from build123d import *

# Parameters (mm, degrees)
SKETCH1_R           = 53.975
SKETCH1_R_2         = 49.975
BOSS_EXTRUDE1_DEPTH = 283.75
SKETCH2_R           = 53.975
BOSS_EXTRUDE2_DEPTH = 4
FILLET1_R           = 5


with BuildPart() as part:
    # Sketch1 → Boss-Extrude1 (new, symmetric)
    with BuildSketch(Plane(origin=(0, 0, 0), x_dir=(1, 0, 0), z_dir=(0, 1, 0))):
        with Locations(Location((0, 0, 0), (0, 0, 270))):
            Circle(SKETCH1_R)
        with Locations(Location((0, 0, 0), (0, 0, 270))):
            Circle(SKETCH1_R_2, mode=Mode.SUBTRACT)
    extrude(amount=BOSS_EXTRUDE1_DEPTH, both=True)

    # Sketch2 → Boss-Extrude2 (add)
    with BuildSketch(Plane.XZ.offset(283.75)):
        with Locations(Location((0, 0, 0), (0, 0, 270))):
            Circle(SKETCH2_R)
    extrude(amount=BOSS_EXTRUDE2_DEPTH)

    # Sketch3 → Revolve1 (revolve)
    with BuildSketch(Plane.XY, mode=Mode.PRIVATE) as revolve1_sk:
        with BuildLine():
            Line((-14.520190182, 339.3125), (-14.520190182, 361.5375))
            Line((-14.520190182, 361.5375), (-10.520190182, 361.5375))
            Line((-10.520190182, 361.5375), (-10.520190182, 336.395540435))
            ThreePointArc((-10.520190182, 336.395540435), (-39.016633765, 316.644661214), (-49.975, 283.75))
            Line((-49.975, 283.75), (-53.975, 283.75))
            ThreePointArc((-53.975, 283.75), (-43.107974032, 317.822985722), (-14.520190182, 339.3125))
        make_face()
    revolve(revolve1_sk.sketch.rotate(Axis((0, 0, 0), (0, 1, 0)), 270), axis=Axis((0, 0, 0), (0, 1, 0)))

    # Fillet1
    fillet1_edges = [part.edges().sort_by_distance(p)[0] for p in [
        (0, -287.75, 53.975),
        (0, 339.3125, 14.520190182),
        (0, -283.75, -49.975),
    ]]
    fillet(fillet1_edges, radius=FILLET1_R)


solid = part.part
Source: CAD feature listing. Evaluate the final solid. Frame: model axes, mm. A direction names the side the tool comes from. Coordinates: 2 decimals unless noted, no trailing zeros. Loops run counter-clockwise (first coordinate to the right, second up) from the corner with the lowest first, then second, coordinate; pieces in that order, holes last. Notation, with made-up numbers: (59, 46.25) -> (76, 46.25) arc R24 cw to (76, 72.25) -> close; hole circle Ø5 at (86, 80). An arc over 180 degrees is marked (long way). Answer in a Markdown table with one row per item. Add a question column.
Q1. Pull-direction query (Z, two-part tool) for faces 4 (the face through (-45.51, 4.47, 29.02)), 5 (the face through (1, -283.75, 1)), 6 (the face through (-4, 361.538, -10)); classes: pulls with the +Z half, pulls with the -Z half, needs draft (parallel to the pull), parting line crosses it, or undercut.
Q2. Contact query for flat-ended pins moving along their axis: pin 1 Ø1.5 at (y, z) = (18.5, -33) entering from +X; pin 2 Ø5 at (x, z) = (-39, -33.5) entering from +Y; pin 3 Ø4 at (x, y) = (20.5, 200.5) entering from +Z. Output: stop coordinate, or through.
Q3. Section A-A on y = -232.5. Return the cut outline in (x, z) (3 decimals).
Q4. Ray query, line 1 along X through (y, z) = (99, 0) (3 decimals); line 2 along X through (y, z) = (355.5, 0); line 3 along Y through (x, z) = (-8, 36). Return the intervals inside material, ascending.
Q5. Reachability of faces 1 (the face through (-7, -287.75, 1)), 2 (the face through (-10.43, 348.79, 1.37)), 3 (the face through (-30.41, -1.44, -39.66)) from +Z, -Z, +X, -X, +Y, -Y: full face, straight path, thin tool, end or side. Return the list, or none.
Computed values:
| question | item | result |
|---|---|---|
| 1 | face 4 | parting line crosses it |
| 1 | face 5 | undercut |
| 1 | face 6 | needs draft |
| 2 | pin 1 | stops at x = 43.28 |
| 2 | pin 2 | stops at y = 307.63 |
| 2 | pin 3 | stops at z = 50.71 |
| 3 | outline | circle Ø107.95 at (0, 0); hole circle Ø99.95 at (0, 0) |
| 4 | line 1 | x = -53.975 to -49.975, 49.975 to 53.975 |
| 4 | line 2 | x = -14.52 to -10.52, 10.52 to 14.52 |
| 4 | line 3 | y = -287.75 to -283.75, 319.32 to 325.22 |
| 5 | face 1 | +Z, -Z, +X, -X, -Y |
| 5 | face 2 | +Y |
| 5 | face 3 | none |
